from build123d import *

# Parameters (mm, degrees)
SKETCH2_W                 = 144
SKETCH2_H                 = 52
BOSS_EXTRUDE2_DEPTH       = 64
SKETCH3_W                 = 96
SKETCH3_H                 = 36
CUT_EXTRUDE1_DEPTH        = 64
SKETCH6_R                 = 8
CUT_EXTRUDE5_DEPTH        = 64
CUT_EXTRUDE7_DEPTH        = 160.712241234
CUT_EXTRUDE8_DEPTH        = 100.779757466
FILLET1_R                 = 3
F_1_0MM_DOWEL_HOLE1_D     = 6
F_1_0MM_DOWEL_HOLE1_DEPTH = 10
F_1_0MM_DOWEL_HOLE1_TIP   = 1.732050808
F_1_0MM_DOWEL_HOLE2_D     = 6
F_1_0MM_DOWEL_HOLE2_DEPTH = 10
F_1_0MM_DOWEL_HOLE2_TIP   = 1.732050808


with BuildPart() as part:
    # Sketch2 → Boss-Extrude2 (new body)
    with BuildSketch(Plane.XY):
        Rectangle(SKETCH2_W, SKETCH2_H)
    extrude(amount=BOSS_EXTRUDE2_DEPTH)

    # Sketch3 → Cut-Extrude1 (cut)
    with BuildSketch(Plane.XY.offset(64)):
        with Locations((2, 8)):
            Rectangle(SKETCH3_W, SKETCH3_H)
    extrude(amount=-CUT_EXTRUDE1_DEPTH, mode=Mode.SUBTRACT)

    # Sketch6 → Cut-Extrude5 (cut)
    with BuildSketch(Plane(origin=(72, 0, 0), x_dir=(0, 0, -1), z_dir=(1, 0, 0))):
        Polygon((-64, 26), (-64, -10), (-60, -10), (-46.287322277, 17.202251187), (-41.852369694, 26), align=None)
        with BuildLine():
            Line((0, 26), (-22.4139537, 26))
            Line((-22.4139537, 26), (-19.003189987, 19.331823481))
            ThreePointArc((-19.003189987, 19.331823481), (-17.755283243, 17.286154301), (-16.826882915, 15.077058))
            Line((-16.826882915, 15.077058), (-4, -10))
            Line((-4, -10), (0, -10))
            Line((0, -10), (0, 26))
        make_face()
        with BuildLine():
            Line((-22.4139537, 26), (-32, 26))
            ThreePointArc((-32, 26), (-24.696205633, 24.235680098), (-19.003189987, 19.331823481))
            Line((-19.003189987, 19.331823481), (-22.4139537, 26))
        make_face()
        with BuildLine():
            Line((-41.852369694, 26), (-46.287322277, 17.202251187))
            ThreePointArc((-46.287322277, 17.202251187), (-40.389397505, 23.624170048), (-32, 26))
            Line((-32, 26), (-41.852369694, 26))
        make_face()
        with Locations((-32, 10)):
            Circle(SKETCH6_R)
    extrude(amount=-CUT_EXTRUDE5_DEPTH, mode=Mode.SUBTRACT)

    # Sketch7 → Cut-Extrude7 (cut, through all)
    with BuildSketch(Plane(origin=(72, 0, 0), x_dir=(0, 0, -1), z_dir=(1, 0, 0))):
        Polygon((-40, -10), (-40, -19), (-32, -19), (-24, -19), (-24, -10), align=None)
        Polygon((-48, -19), (-48, -26), (-16, -26), (-16, -19), (-24, -19), (-32, -19), (-40, -19), align=None)
    extrude(amount=-CUT_EXTRUDE7_DEPTH, mode=Mode.SUBTRACT)

    # Sketch8 → Cut-Extrude8 (cut, through all)
    with BuildSketch(Plane.XY.offset(64)):
        Polygon((-72, 26), (-56, 26), (-72, 10), align=None)
    extrude(amount=-CUT_EXTRUDE8_DEPTH, mode=Mode.SUBTRACT)

    # Fillet1
    fillet1_edges = [part.edges().sort_by_distance(p)[0] for p in [
        (61, -10, 4),
        (61, -10, 60),
    ]]
    fillet(fillet1_edges, radius=FILLET1_R)

    # Ø1.0mm Dowel Hole1
    with Locations(Plane(origin=(-36, -26, 56), x_dir=(0, 0, -1), z_dir=(0, -1, 0))):
        with Locations((0, 0), (0, 70)):
            Hole(F_1_0MM_DOWEL_HOLE1_D / 2, depth=F_1_0MM_DOWEL_HOLE1_DEPTH)
            with Locations((0, 0, -(F_1_0MM_DOWEL_HOLE1_DEPTH + F_1_0MM_DOWEL_HOLE1_TIP / 2))):  # 120° drill point
                Cone(0, F_1_0MM_DOWEL_HOLE1_D / 2, F_1_0MM_DOWEL_HOLE1_TIP, mode=Mode.SUBTRACT)

    # Ø1.0mm Dowel Hole2
    with Locations(Plane(origin=(-36, -26, 8), x_dir=(0, 0, -1), z_dir=(0, -1, 0))):
        with Locations((0, 0), (0, 70)):
            Hole(F_1_0MM_DOWEL_HOLE2_D / 2, depth=F_1_0MM_DOWEL_HOLE2_DEPTH)
            with Locations((0, 0, -(F_1_0MM_DOWEL_HOLE2_DEPTH + F_1_0MM_DOWEL_HOLE2_TIP / 2))):  # 120° drill point
                Cone(0, F_1_0MM_DOWEL_HOLE2_D / 2, F_1_0MM_DOWEL_HOLE2_TIP, mode=Mode.SUBTRACT)


solid = part.part
Verification items for the finished model (mm, model axes). A direction names the side the tool comes from. Give positions to 0.01 mm unless a question says otherwise; leave off trailing zeros. Write each loop counter-clockwise with the first axis right and the second up, starting at its lowest first coordinate (ties: lowest second). Pieces come first, ordered by that corner, then holes. Notation, with made-up numbers: (41.25, 79.25) - (75.25, 79.25) arc R17 cw to (75.25, 110.25) - close; hole circle Ø7 at (29, 79.25). An arc over 180 degrees is marked (long way). Answer as CSV lines item,"result". Start each with the question number.
1. Sectioned sample at B-B (y = 4). Record the boundary of the cut face in (x, z), then the cut area to 3 significant figures.
2. Sectioned sample at C-C (x = -50.5). Record the boundary of the cut face in (y, z), then the cut area to 3 significant figures.
3. Draft check along X on faces 6 (the face through (1, -19, 44)), 7 (the face through (-46, 8, 32)), 8 (the face through (-72, -4, 32)). Enter one of: pulls with the +X half, pulls with the -X half, needs draft (parallel to the pull), parting line crosses it, or undercut.
4. Sectioned sample at A-A (x = 3). Record the boundary of the cut face in (y, z), then the cut area to 3 significant figures.
5. Thickness scan on line 1 (X direction, y = -19.5, z = 56); line 2 (Z direction, x = 34, y = -18); line 3 (Z direction, x = 34, y = -23.25). Record the ranges inside material, lowest first.
6. Depth check by flat-ended pin: pin 1 (6.5 mm diameter, centred on x = 10.5, z = 44.5, fed in from -Y); pin 2 (12 mm diameter, centred on x = 7, z = 51.5, fed in from +Y); pin 3 (8 mm diameter, centred on x = -56.5, z = 29, fed in from -Y). Enter the tip coordinate at first touch or a pass-through.
7. Set-up check for faces 1 (the face through (-1, -26, 56)), 2 (the face through (36.53, -20.93, 9.61)), 3 (the face through (60.846, -9.567, 60.294)), 4 (the face through (1, -14, 40)), 5 (the face through (61.154, 3.52, 10.915)): record each of +Z, -Z, +X, -X, +Y, -Y from which the full face is reachable in a straight line by a thin tool's end or side.
Derived:
1,outline,"(-72, 0) - (-46, 0) - (-46, 64) - (-72, 64) - close; (50, 11.16) - (72, 11.16) - (72, 26.71) - (50, 26.71) - close; (50, 37.29) - (72, 37.29) - (72, 52.94) - (50, 52.94) - close"
1,area,"2,350 mm²"
2,outline,"(-26, 0) - (26, 0) - (26, 64) - (-26, 64) - (-26, 48) - (-19, 48) - (-19, 40) - (-10, 40) - (-10, 24) - (-19, 24) - (-19, 16) - (-26, 16) - close"
2,area,"2,960 mm²"
3,face 6,"needs draft"
3,face 7,"undercut"
3,face 8,"pulls with the -X half"
4,outline,"(-26, 0) - (-10, 0) - (-10, 24) - (-19, 24) - (-19, 16) - (-26, 16) - close; (-26, 48) - (-19, 48) - (-19, 40) - (-10, 40) - (-10, 64) - (-26, 64) - close"
4,area,"656 mm²"
5,line 1,"-72 to -39, -33 to 31, 37 to 72"
5,line 2,"0 to 5, 11 to 24, 40 to 53, 59 to 64"
5,line 3,"0 to 5, 11 to 16, 48 to 53, 59 to 64"
6,pin 1,"y = -19"
6,pin 2,"y = -10"
6,pin 3,"y = -10"
7,face 1,"+Z, -Z, +X, -X, -Y"
7,face 2,"-Y"
7,face 3,"+Z, +X, +Y"
7,face 4,"+X, -X, -Y"
7,face 5,"-Z, +X, +Y"
